```python
from build123d import *

# Parameters (mm, degrees)
BOSS_EXTRUDE1_DEPTH          = 50.8
F_1_8_0_125_DIAMETER_HOLE1_D = 3.175
FILLET2_R                    = 3.175


with BuildPart() as part:
    # Sketch1 → Boss-Extrude1 (new body)
    with BuildSketch(Plane.XY):
        Polygon((17.4625, 9.525), (17.4625, 1.5875), (1.5875, 1.5875), (1.5875, 9.525), (0, 9.525), (0, 0), (19.05, 0), (19.05, 9.525), align=None)
    extrude(amount=BOSS_EXTRUDE1_DEPTH)

    # 1/8 (0.125) Diameter Hole1 (through all)
    with Locations(Plane(origin=(19.05, 0, 0), x_dir=(0, 0, -1), z_dir=(1, 0, 0))):
        with Locations((-3.175, 6.35)):
            Hole(F_1_8_0_125_DIAMETER_HOLE1_D / 2)

    # Fillet2
    fillet2_edges = [part.edges().sort_by_distance(p)[0] for p in [
        (0.79375, 9.525, 0),
        (18.25625, 9.525, 0),
    ]]
    fillet(fillet2_edges, radius=FILLET2_R)


solid = part.part
```
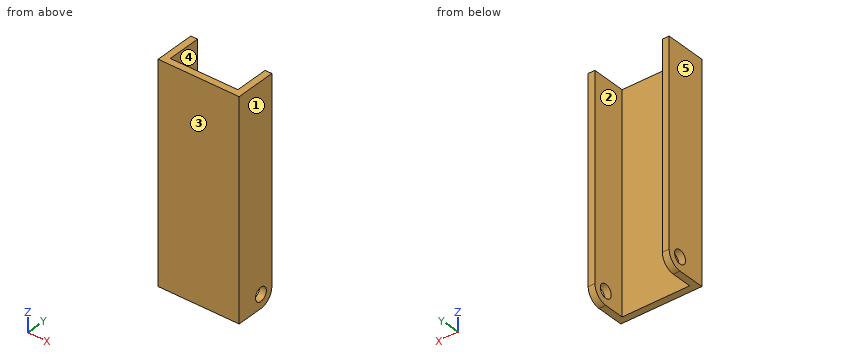
Can you work these out from the model? Positions are in its coordinate system, mm. Face numbers are marked on the shaded views. A direction names the side the tool comes from. Coordinates: 2 decimals unless noted, no trailing zeros. Loops run counter-clockwise (first coordinate to the right, second up) from the corner with the lowest first, then second, coordinate; pieces in that order, holes last. Notation, with made-up numbers: M -33.75,64.25 L -18.75,64.25 A29 cw -18.75,97.25 Z; hole C 61.5,-29 d7. An arc over 180 degrees is marked long. Put each result on its own line as item: value. Start each with the question number.
(1) Will these pins go through, and if not, where does the flat tip stop? pin 1 Ø4 at (x, z) = (7, 41.5) entering from +Y; pin 2 Ø2.5 at (y, z) = (6.35, 3.175) entering from +X; pin 3 Ø2 at (y, z) = (8, 12) entering from -X.
(2) I need wall thicknesses on probe 1 along X at (y, z) = (4.5, 4.5); probe 2 along Y at (x, z) = (3.5, 25); probe 3 along Y at (x, z) = (18, 3.5) (3 decimals). Which ranges of each line are inside material? Lowest first, please.
(3) Imagine slicing it at C-C on x = 8.25. List the corners of the cut face in (y, z) for me, and give its area (3 significant figures).
(4) We'd pull the mould along X, two halves only. Please class the marked faces 1, 2 and 3: +X half, -X half, draft (parallel to the pull), parting line (faces both ways), or undercut.
(5) Which directions (+Z, -Z, +X, -X, +Y, -Y) give clear straight access to the entire face, cutting with the end or side of a thin tool? Please do the marked faces 4 and 5.
(6) Imagine slicing it at B-B on y = 7. List the corners of the cut face in (x, z) for me, and give its area (3 significant figures).
Worked answers:
1. pin 1: stops at y = 1.59
1. pin 2: passes through
1. pin 3: stops at x = 0
2. probe 1: x = 0 to 1.59, 17.46 to 19.05
2. probe 2: y = 0 to 1.59
2. probe 3: y = 0 to 4.796, 7.904 to 9.525
3. outline: M 0,0 L 1.59,0 L 1.59,50.8 L 0,50.8 Z
3. area: 80.6 mm2
4. face 1: +X half
4. face 2: undercut
4. face 3: draft
5. face 4: +Z, -Z, +Y
5. face 5: +Z, -Z, -X, +Y, -Y
6. outline: M 0,0.07 L 1.59,0.07 L 1.59,1.73 L 0,1.73 Z; M 0,4.62 L 1.59,4.62 L 1.59,50.8 L 0,50.8 Z; M 17.46,0.07 L 19.05,0.07 L 19.05,1.73 L 17.46,1.73 Z; M 17.46,4.62 L 19.05,4.62 L 19.05,50.8 L 17.46,50.8 Z
6. area: 152 mm2
